```python
from build123d import *

# Parameters (mm, degrees)
SKETCH1_R           = 1.7145
MAINBODY_DEPTH      = 1.2
LARGEROUNDS_R       = 7.5184
SMALLROUNDS_R       = 1.5748
PCBMOUNTHOLES_REACH = 82.573
SKETCH2_R           = 1.345


with BuildPart() as part:
    # Sketch1 → MainBody (new body)
    with BuildSketch(Plane.XY):
        Polygon((71.6788, -27.4828), (71.6788, 27.4828), (53.1114, 27.4828), (53.1114, 36.7792), (18.5674, 36.7792), (18.5674, 27.4828), (0, 27.4828), (0, -27.4828), (18.5674, -27.4828), (18.5674, -36.7792), (53.1114, -36.7792), (53.1114, -27.4828), align=None)
        with Locations((64.8462, -21.7424)):
            Circle(SKETCH1_R, mode=Mode.SUBTRACT)
        with Locations(Location((6.8326, -21.7424, 0), (0, 0, 180))):
            Circle(SKETCH1_R, mode=Mode.SUBTRACT)
        with Locations((6.8326, 21.7424)):
            Circle(SKETCH1_R, mode=Mode.SUBTRACT)
        with Locations(Location((64.8462, 21.7424, 0), (0, 0, 180))):
            Circle(SKETCH1_R, mode=Mode.SUBTRACT)
        with Locations((35.8394, -28.8671)):
            Circle(SKETCH1_R, mode=Mode.SUBTRACT)
        with Locations(Location((35.8394, 28.8671, 0), (0, 0, 180))):
            Circle(SKETCH1_R, mode=Mode.SUBTRACT)
    extrude(amount=MAINBODY_DEPTH)

    # LargeRounds
    largerounds_edges = [part.edges().sort_by_distance(p)[0] for p in [
        (53.1114, -27.4828, 0.6),
        (18.5674, -27.4828, 0.6),
        (18.5674, 27.4828, 0.6),
        (53.1114, 27.4828, 0.6),
    ]]
    fillet(largerounds_edges, radius=LARGEROUNDS_R)

    # SmallRounds
    smallrounds_edges = [part.edges().sort_by_distance(p)[0] for p in [
        (53.1114, -36.7792, 0.6),
        (18.5674, -36.7792, 0.6),
        (0, -27.4828, 0.6),
        (0, 27.4828, 0.6),
        (18.5674, 36.7792, 0.6),
        (53.1114, 36.7792, 0.6),
        (71.6788, 27.4828, 0.6),
        (71.6788, -27.4828, 0.6),
    ]]
    fillet(smallrounds_edges, radius=SMALLROUNDS_R)

    # Sketch2 → PCBMountHoles (cut, up to next)
    with BuildSketch(Plane.XY.offset(1.2), mode=Mode.PRIVATE) as pcbmountholes_sk1:
        with Locations((30.7594, -16.76)):
            Circle(SKETCH2_R)
    pcbmountholes_tool1 = extrude(pcbmountholes_sk1.sketch, amount=-PCBMOUNTHOLES_REACH, mode=Mode.PRIVATE) & part.part
    # Sketch2 → PCBMountHoles (cut, up to next)
    with BuildSketch(Plane.XY.offset(1.2), mode=Mode.PRIVATE) as pcbmountholes_sk2:
        with Locations((43.0794, -16.76)):
            Circle(SKETCH2_R)
    pcbmountholes_tool2 = extrude(pcbmountholes_sk2.sketch, amount=-PCBMOUNTHOLES_REACH, mode=Mode.PRIVATE) & part.part
    # Sketch2 → PCBMountHoles (cut, up to next)
    with BuildSketch(Plane.XY.offset(1.2), mode=Mode.PRIVATE) as pcbmountholes_sk3:
        with Locations((43.0794, 18.02)):
            Circle(SKETCH2_R)
    pcbmountholes_tool3 = extrude(pcbmountholes_sk3.sketch, amount=-PCBMOUNTHOLES_REACH, mode=Mode.PRIVATE) & part.part
    add(pcbmountholes_tool1.solids().sort_by_distance((30.7594, -16.76, 1.2))[0], mode=Mode.SUBTRACT)
    add(pcbmountholes_tool2.solids().sort_by_distance((43.0794, -16.76, 1.2))[0], mode=Mode.SUBTRACT)
    add(pcbmountholes_tool3.solids().sort_by_distance((43.0794, 18.02, 1.2))[0], mode=Mode.SUBTRACT)


solid = part.part
```
Here's how the part is built. I have some questions about the finished solid (model axes, mm). Coordinates: 2 decimals unless noted, no trailing zeros. Write each loop counter-clockwise with the first axis right and the second up, starting at its lowest first coordinate (ties: lowest second). Pieces come first, ordered by that corner, then holes. Notation, with made-up numbers: (-12.5, 24.5) -> (9.5, 24.5) arc R22 ccw to (9.5, 37.5) -> close; hole circle Ø9 at (11, 59). An arc over 180 degrees is marked (long way). Use a Markdown table: item, result. Add a question column.
(1) I'm going to push flat-ended pins straight in: P1, Ø2, axis at x = 43.08, y = -16.76, coming from the +Z side; P2, Ø0.6, axis at x = 6.5, z = 0.5, coming from the -Y side. Where does each tip first touch, or does it pass through?
(2) If we section it at D-D, the plane z = 0.9: State how many separate pieces and enclosed holes the cut face has, and give its area (3 significant figures).
(3) If we section it at A-A, the plane y = -16.76: Write out the boundary of the cut face in (x, z).
(4) If we section it at C-C, the plane x = 7: Write out the boundary of the cut face in (y, z).
(5) Please list where these lines run through material, in increasing order: line 1 (Y direction, x = 7, z = 0.25); line 2 (Y direction, x = 43, z = 0.25); line 3 (Y direction, x = 63, z = 0.25).
(6) If we section it at B-B, the plane y = 18.02: Write out the boundary of the cut face in (x, z), and give its area (3 significant figures).
(7) We'd pull the mould along Y, two halves only. Please class faces 1 (the cylindrical face through (37.475, -28.352, 0.592)), 2 (the cylindrical face through (0.47, -27.03, 0.61)), 3 (the cylindrical face through (52.66, 36.31, 0.61)): +Y half, -Y half, draft (parallel to the pull), parting line (faces both ways), or undercut.
Outcome:
| question | item | result |
|---|---|---|
| 1 | P1 | passes through |
| 1 | P2 | stops at y = -27.48 |
| 2 | separate pieces | 1 |
| 2 | enclosed holes | 9 |
| 2 | area | 4,550 mm^2 |
| 3 | outline | (0, 0) -> (29.41, 0) -> (29.41, 1.2) -> (0, 1.2) -> close; (32.1, 0) -> (41.73, 0) -> (41.73, 1.2) -> (32.1, 1.2) -> close; (44.42, 0) -> (71.68, 0) -> (71.68, 1.2) -> (44.42, 1.2) -> close |
| 4 | outline | (-27.48, 0) -> (-23.45, 0) -> (-23.45, 1.2) -> (-27.48, 1.2) -> close; (-20.04, 0) -> (20.04, 0) -> (20.04, 1.2) -> (-20.04, 1.2) -> close; (23.45, 0) -> (27.48, 0) -> (27.48, 1.2) -> (23.45, 1.2) -> close |
| 5 | line 1 | y = -27.48 to -23.45, -20.04 to 20.04, 23.45 to 27.48 |
| 5 | line 2 | y = -36.78 to -18.1, -15.42 to 16.68, 19.36 to 36.78 |
| 5 | line 3 | y = -27.48 to 27.48 |
| 6 | outline | (0, 0) -> (41.73, 0) -> (41.73, 1.2) -> (0, 1.2) -> close; (44.42, 0) -> (71.68, 0) -> (71.68, 1.2) -> (44.42, 1.2) -> close |
| 6 | area | 82.8 mm^2 |
| 7 | face 1 | undercut |
| 7 | face 2 | -Y half |
| 7 | face 3 | +Y half |
